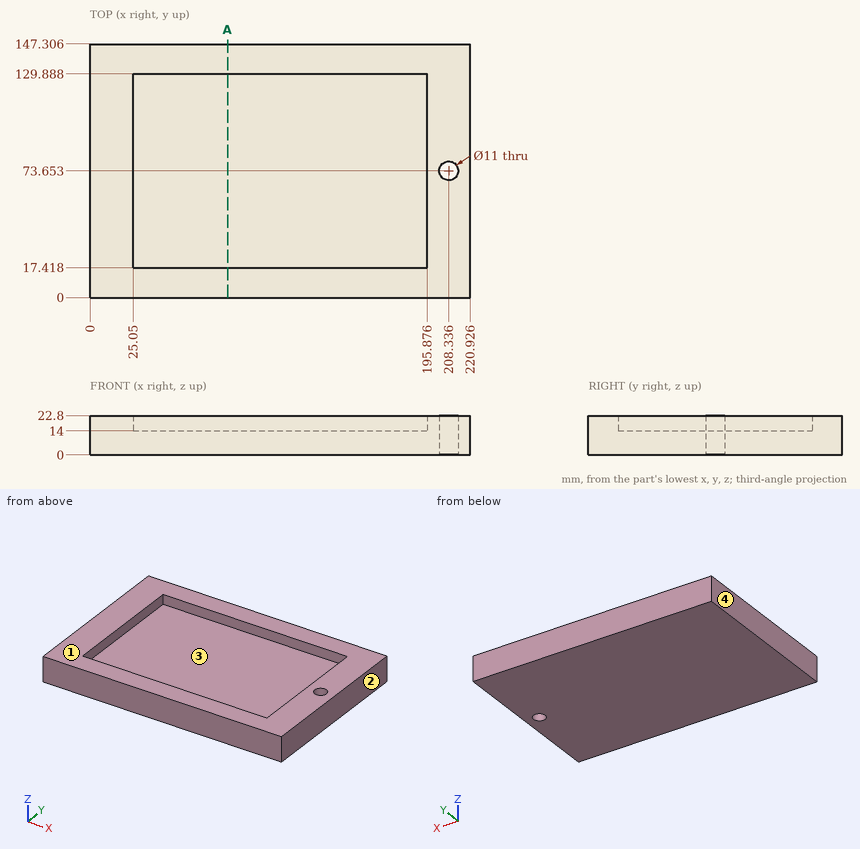
Design review of the part shown in the three views and the two pictorial views. Dimensions are in mm from the part's minimum x, y and z. Round coordinates to 2 decimals unless told otherwise and drop trailing zeros. Write each loop counter-clockwise with the first axis right and the second up, starting at its lowest first coordinate (ties: lowest second). Pieces come first, ordered by that corner, then holes. Notation, with made-up numbers: (-23, -19) - (17, -19) arc R16 cw to (17, 11) - close; hole circle Ø2 at (40.5, -9.75). An arc over 180 degrees is marked (long way). Write item = value, one per line. Start each with the question number.
1. Draft analysis for pull direction X (two halves, no side actions). For the marked faces 1, 2, 3 and 4, state which applies: released by +X, released by -X, zero draft, split by the parting line, or undercut.
2. Wall thickness on L1, parallel to Y at x = 122.5, z = 16.25 (1 decimal); L2, parallel to Z at x = 126, y = 91; L3, parallel to Y at x = 207.5, z = 16 (1 decimal): over which ranges is each line inside the solid? List them lowest first.
3. For pin 1 Ø1 at (x, y) = (131.5, 37.5) entering from +Z; pin 2 Ø4 at (y, z) = (61, 4.5) entering from -X, all flat-tipped, find the tip position at first contact; note any pin that passes through.
4. Consider section A-A on x = 80. State the section outline as (y, z) points (1 decimal), plus the area to 3 significant figures.
Evaluation:
q1.face_1 = zero draft
q1.face_2 = released by +X
q1.face_3 = undercut
q1.face_4 = released by -X
q2.L1 = 0 to 17.4, 129.9 to 147.3
q2.L2 = 0 to 14
q2.L3 = 0 to 68.2, 79.1 to 147.3
q3.pin_1 = 14
q3.pin_2 = 0
q4.outline = (0, 0) - (147.3, 0) - (147.3, 22.8) - (129.9, 22.8) - (129.9, 14) - (17.4, 14) - (17.4, 22.8) - (0, 22.8) - close
q4.area = 2,370 mm2
